Geometry: final body of the model. Coordinates: model frame, mm. Face numbers are marked on the shaded views. A direction names the side the tool comes from. Give positions to 0.01 mm unless a question says otherwise; leave off trailing zeros. Write each loop counter-clockwise with the first axis right and the second up, starting at its lowest first coordinate (ties: lowest second). Pieces come first, ordered by that corner, then holes.
Q1. Cut plane A-A on y = 0. Return the cut outline in (x, z), plus the area to 3 significant figures.
Q2. Draft query along Y for the marked faces 4, 5 and 6. Return one class per face: pulls with the +Y half, pulls with the -Y half, needs draft (parallel to the pull), parting line crosses it, or undercut.
Q3. Cut plane C-C on z = 1.5. Return the cut outline in (x, y).
Q4. Pin query (flat end, axial travel): pin 1 (1.5 mm diameter, centred on y = 0.5, z = -5.5, fed in from -X); pin 2 (2 mm diameter, centred on x = -2, z = -0.5, fed in from -Y). Return the tip coordinate at first contact, or that it passes through.
Q5. Cut plane B-B on z = -4.5. Return the cut outline in (x, y).
Q6. Line query: L1, parallel to Z at x = 1.6, y = -1.6; L2, parallel to Z at x = -0.9, y = -0.05; L3, parallel to Y at x = -0.05, z = -2. Output: solid intervals per line, ascending.
Q7. Reachability of the marked faces 1, 2 and 3 from +Z, -Z, +X, -X, +Y, -Y: full face, straight path, thin tool, end or side. Return the list, or none.
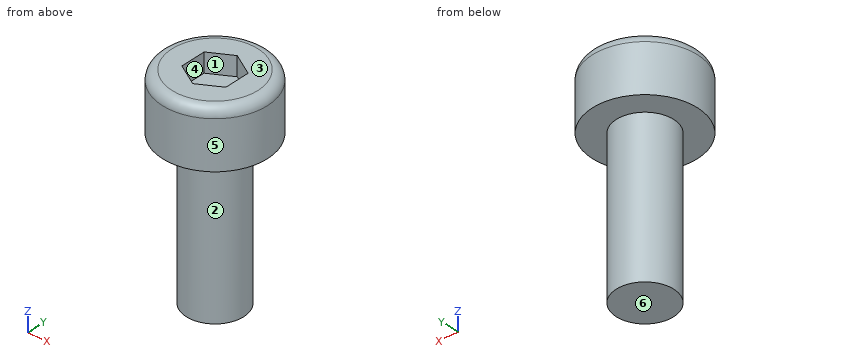
Autodesk Inventor part; units mm, degrees
ref_plane "YZ Plane" through (0, 0, 0) normal (1, 0, 0) x (0, 1, 0)
ref_plane "XZ Plane" through (0, 0, 0) normal (0, 1, 0) x (-1, 0, 0)
ref_plane "XY Plane" through (0, 0, 0) normal (0, 0, 1) x (1, 0, 0)
sketch "Sketch3" plane through (0, 0, 0) normal (0, 0, 1) x (1, 0, 0)
  circle A0 centre (0, 0) radius 2.75
  circle A1 centre (0, 0) radius 1.5
  line L0 (1.15, -0.664) -> (0, -1.3279)
  line L1 (0, -1.3279) -> (-1.15, -0.664)
  line L2 (-1.15, -0.664) -> (-1.15, 0.664)
  line L3 (-1.15, 0.664) -> (0, 1.3279)
  line L4 (0, 1.3279) -> (1.15, 0.664)
  line L5 (1.15, 0.664) -> (1.15, -0.664)
  point P0 (1.15, 0)
  dimension "d8" = 1.5
  dimension "d9" = 2.75
  dimension "d10" = 2.3
extrude "Extrusion1" add sketch "Sketch3" along normal blind 3 contours A0 | A1 | L0 L1 L2 L3 L4 L5
extrude "Extrusion2" add sketch "Sketch3" against normal blind 8 contours A1 | L0 L1 L2 L3 L4 L5
extrude "Extrusion3" cut sketch "Sketch3" against normal blind 1 from surface at 3 contours L0 L1 L2 L3 L4 L5
fillet "Fillet1" radius 0.5 1 edges at (-2.75, 0, 3)
thread "Thread2"
properties part number "MachineScrew_Template"
Data:
1. outline: (-2.75, 0) - (-1.5, 0) - (-1.5, -8) - (1.5, -8) - (1.5, 0) - (2.75, 0) - (2.75, 2.5) arc R0.5 ccw to (2.25, 3) - (1.15, 3) - (1.15, 2) - (-1.15, 2) - (-1.15, 3) - (-2.25, 3) arc R0.5 ccw to (-2.75, 2.5) - close
1. area: 38.1 mm2
2. face 4: undercut
2. face 5: parting line crosses it
2. face 6: needs draft
3. outline: circle Ø5.5 at (0, 0)
4. pin 1: stops at x = -1.5
4. pin 2: stops at y = -2.51
5. outline: circle Ø3 at (0, 0)
6. L1: z = 0 to 3
6. L2: z = -8 to 2
6. L3: y = -1.5 to 1.5
7. face 1: +Z
7. face 2: -Z
7. face 3: +Z, +X, -X, +Y, -Y
